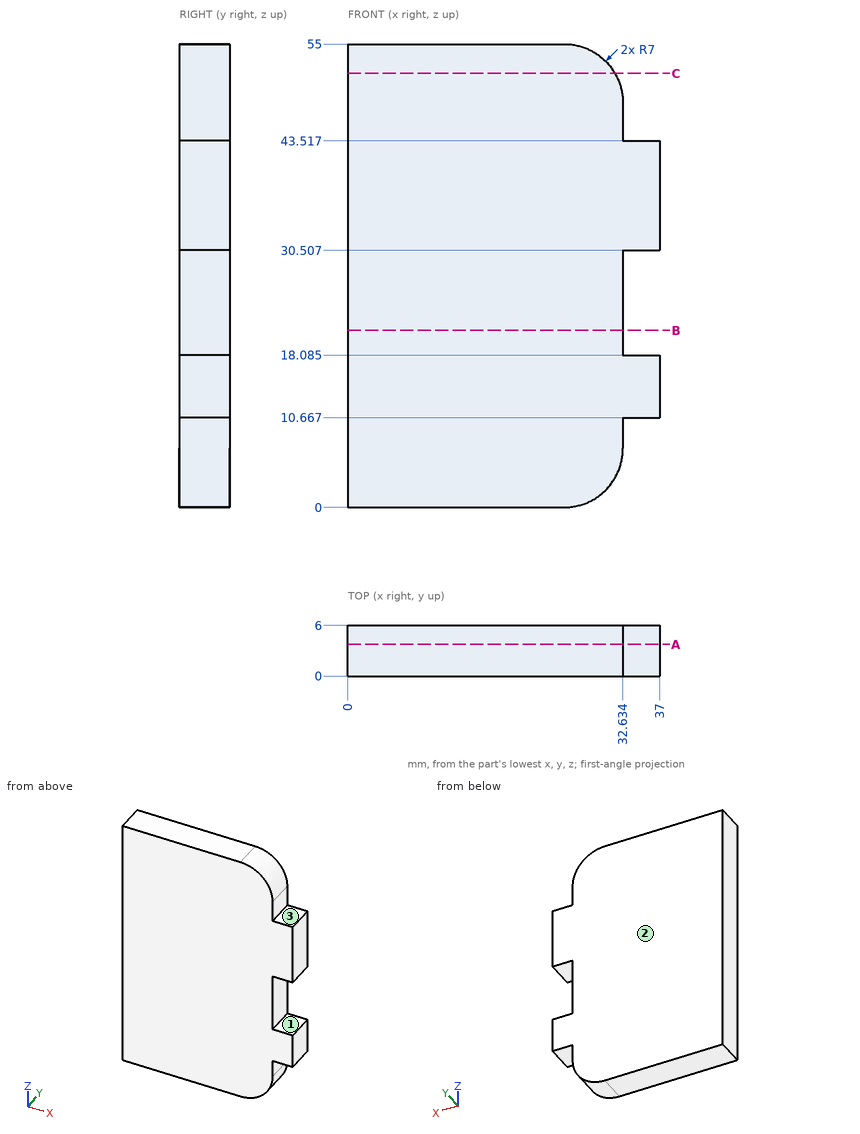
Check sheet for the drawn part. Datum: minimum x, y, z corner. Units: mm. A direction names the side the tool comes from. Round coordinates to 2 decimals unless told otherwise and drop trailing zeros. Write each loop counter-clockwise with the first axis right and the second up, starting at its lowest first coordinate (ties: lowest second). Pieces come first, ordered by that corner, then holes. Notation, with made-up numbers: (-37, -38) -> (4, -38) arc R10 ccw to (4, -21) -> close; hole circle Ø3 at (70, 14.25). An arc over 180 degrees is marked (long way). One line per item, written item: value. Start each with the question number.
(1) Scan lines: line 1 (X direction, y = 3.8, z = 9.5); line 2 (X direction, y = 3.9, z = 5); line 3 (Z direction, x = 32, y = 2.9) (1 decimal). Record each from-to range of solid material in increasing order. Write a range as [from, to].
(2) Cross-section at B-B, the plane z = 21. Record the cut outline in (x, y), and give its area (3 significant figures).
(3) Cross-section at C-C, the plane z = 51.5. Record the cut outline in (x, y).
(4) Cross-section at A-A, the plane y = 3.75. Record the cut outline in (x, z) (1 decimal), and give its area (3 significant figures).
(5) Go/stop test with flat-tipped pins: pin 1 Ø1.3 at (x, y) = (34, 4) entering from -Z; pin 2 Ø3 at (y, z) = (5, 45) entering from -X; pin 3 Ø3.5 at (x, y) = (35.5, 1.5) entering from +Z; pin 4 Ø1.1 at (y, z) = (4, 8) entering from +X. Record where each tip stops, or that it passes through.
(6) Access from +Z, -Z, +X, -X, +Y, -Y to the whole of each face (thin tool, end or side, straight path). Record for the marked faces 1, 2 and 3.
Answer:
1. line 1: [0, 32.63]
1. line 2: [0, 32.34]
1. line 3: [4.1, 50.9]
2. outline: (0, 0) -> (32.63, 0) -> (32.63, 6) -> (0, 6) -> close
2. area: 196 mm²
3. outline: (0, 0) -> (31.7, 0) -> (31.7, 6) -> (0, 6) -> close
4. outline: (0, 0) -> (25.6, 0) arc R7 ccw to (32.6, 7) -> (32.6, 10.7) -> (37, 10.7) -> (37, 18.1) -> (32.6, 18.1) -> (32.6, 30.5) -> (37, 30.5) -> (37, 43.5) -> (32.6, 43.5) -> (32.6, 48) arc R7 ccw to (25.6, 55) -> (0, 55) -> close
4. area: 1,860 mm²
5. pin 1: z = 10.67
5. pin 2: x = 0
5. pin 3: z = 43.52
5. pin 4: x = 32.63
6. face 1: +X, +Y, -Y
6. face 2: +Z, -Z, +X, -X, +Y
6. face 3: +Z, +X, +Y, -Y
